Read the model definition and answer for the solid it produces. Units are mm, in the model's axes. Give positions to 0.01 mm unless a question says otherwise; leave off trailing zeros. Order: outer loops, then holes, each group sorted by start corner. A loop starts at its lowest first (then second) coordinate and runs counter-clockwise, first axis right, second up. Notation, with made-up numbers: M 23.25,-12.75 L 27.25,-12.75 A22 ccw 27.25,18.25 Z; hole C 4,86 d1. An arc over 180 degrees is marked long. One line per item, written item: value.
from build123d import *

# Parameters (mm, degrees)
SKETCH1_W           = 21.1074
SKETCH1_H           = 15.748
SKETCH1_R           = 1.55575
SKETCH1_R_2         = 0.508
BOSS_EXTRUDE1_DEPTH = 0.5715


with BuildPart() as part:
    # Sketch1 → Boss-Extrude1 (new body, symmetric)
    with BuildSketch(Plane(origin=(0, 0, 0), x_dir=(1, 0, 0), z_dir=(0, 1, 0))):
        Rectangle(SKETCH1_W, SKETCH1_H)
        with Locations((-7.77875, -5.23875)):
            Circle(SKETCH1_R, mode=Mode.SUBTRACT)
        with Locations((7.77875, -5.23875)):
            Circle(SKETCH1_R, mode=Mode.SUBTRACT)
        with Locations((-9.0043, 6.731)):
            Circle(SKETCH1_R_2, mode=Mode.SUBTRACT)
        with Locations((-6.4643, 6.731)):
            Circle(SKETCH1_R_2, mode=Mode.SUBTRACT)
        with Locations((-3.9243, 6.731)):
            Circle(SKETCH1_R_2, mode=Mode.SUBTRACT)
        with Locations((-1.3843, 6.731)):
            Circle(SKETCH1_R_2, mode=Mode.SUBTRACT)
        with Locations((1.1557, 6.731)):
            Circle(SKETCH1_R_2, mode=Mode.SUBTRACT)
        with Locations((3.6957, 6.731)):
            Circle(SKETCH1_R_2, mode=Mode.SUBTRACT)
        with Locations((6.2357, 6.731)):
            Circle(SKETCH1_R_2, mode=Mode.SUBTRACT)
        with Locations((8.7757, 6.731)):
            Circle(SKETCH1_R_2, mode=Mode.SUBTRACT)
    extrude(amount=BOSS_EXTRUDE1_DEPTH, both=True)


solid = part.part
1) Determine the mould class of faces 1 (the face through (0, 0, 7.874)), 2 (the face through (-8.52, -0.01, -6.88)), 3 (the face through (10.554, 0, 0)) for opening direction X: +X half, -X half, draft (parallel to the pull), parting line (faces both ways), or undercut.
Reported:
face 1: draft
face 2: undercut
face 3: +X half
2) Find section B-B, the plane y = -0.2. Count the separate pieces of the cut face and the enclosed holes in it, plus the area to 3 significant figures.
Reported:
separate pieces: 1
enclosed holes: 10
area: 311 mm^2
3) Consider probe 1 along Z at (x, y) = (7.75, 0.4); probe 2 along Z at (x, y) = (8.5, -0.4); probe 3 along X at (y, z) = (-0.2, 4). Determine where each line is inside the solid, lowest interval first.
Reported:
probe 1: z = -7.87 to 3.68, 6.79 to 7.87
probe 2: z = -7.87 to -7.16, -6.3 to 3.86, 6.62 to 7.87
probe 3: x = -10.55 to -8.72, -6.84 to 6.84, 8.72 to 10.55
4) Find section C-C, the plane z = 6. Write down the section's boundary in (x, y), plus the area to 3 significant figures.
Reported:
outline: M -10.55,-0.57 L -9.14,-0.57 L -9.14,0.57 L -10.55,0.57 Z; M -6.42,-0.57 L 6.42,-0.57 L 6.42,0.57 L -6.42,0.57 Z; M 9.14,-0.57 L 10.55,-0.57 L 10.55,0.57 L 9.14,0.57 Z
area: 17.9 mm^2
5) Find section A-A, the plane x = -7.5. Write down the section's boundary in (y, z), plus the area to 3 significant figures.
Reported:
outline: M -0.57,-7.87 L 0.57,-7.87 L 0.57,3.71 L -0.57,3.71 Z; M -0.57,6.77 L 0.57,6.77 L 0.57,7.87 L -0.57,7.87 Z
area: 14.5 mm^2
6) Find section D-D, the plane x = 7. Write down the section's boundary in (y, z), plus the area to 3 significant figures.
Reported:
outline: M -0.57,-7.87 L 0.57,-7.87 L 0.57,3.89 L -0.57,3.89 Z; M -0.57,6.59 L 0.57,6.59 L 0.57,7.87 L -0.57,7.87 Z
area: 14.9 mm^2
